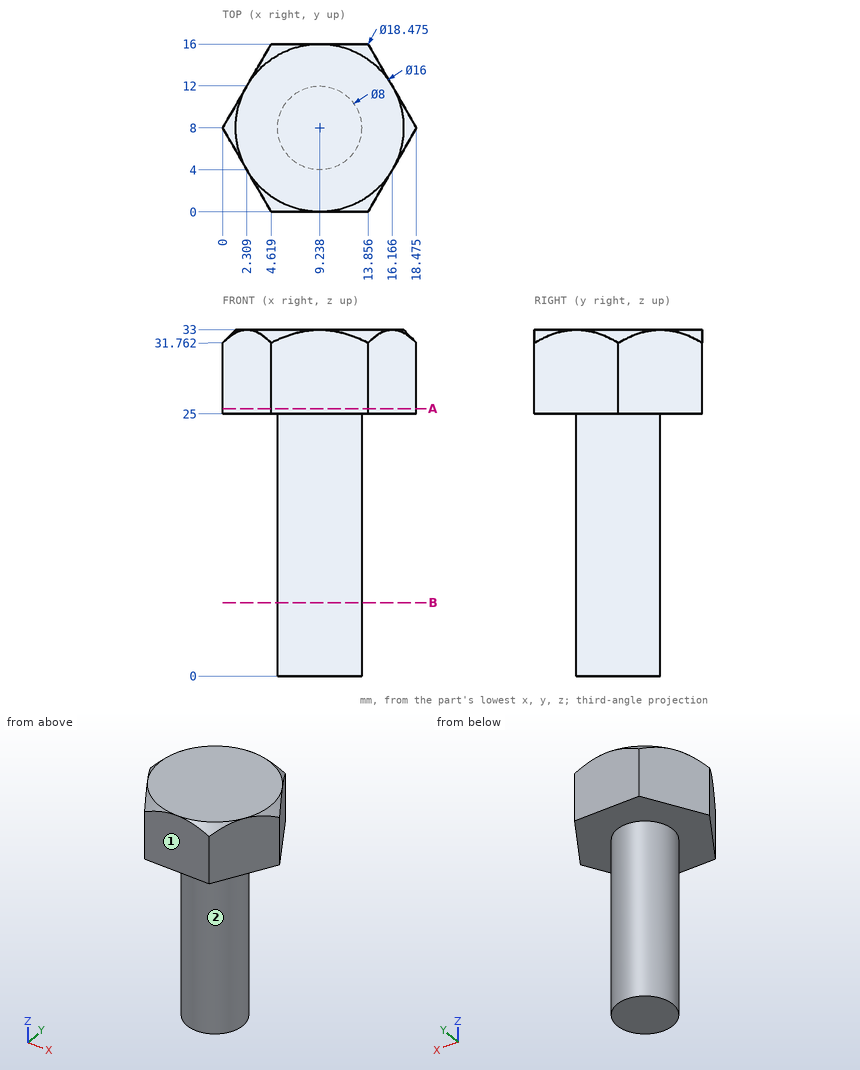
Input: dimensioned drawing with shaded views. Units: mm. Origin: part minimum x, y, z. A direction names the side the tool comes from. Coordinates: 2 decimals unless noted, no trailing zeros. Order: outer loops, then holes, each group sorted by start corner. A loop starts at its lowest first (then second) coordinate and runs counter-clockwise, first axis right, second up.
1. Cut plane B-B, the plane z = 7. Return loops of the section in (x, y).
Checked values:
outline: circle Ø8 at (9.24, 8)
2. Contact query for flat-ended pins moving along their axis: P1, Ø8, axis at y = 8.5, z = 27, coming from the -X side; P2, Ø6, axis at x = 2.5, y = 11.5, coming from the -Z side; P3, Ø2, axis at y = 4, z = 23.5, coming from the -X side; P4, Ø8, axis at y = 5.5, z = 11.5, coming from the +X side. Output: stop coordinate, or through.
Checked values:
P1: stops at x = 0
P2: stops at z = 25
P3: stops at x = 6.59
P4: stops at x = 13.24
3. Cut plane A-A, the plane z = 25.5. Return loops of the section in (x, y) (1 decimal).
Checked values:
outline: (0, 8) - (4.6, 0) - (13.9, 0) - (18.5, 8) - (13.9, 16) - (4.6, 16) - close
4. Access query for the marked faces 1 and 2. Directions: +Z, -Z, +X, -X, +Y, -Y. A direction counts if a zero-diameter tool reaches every point of the face in a straight line with its end or side. Return the directions, or none.
Checked values:
face 1: +Z, -Z, +X, -X, -Y
face 2: -Z
5. Ray query, line 1 along Z through (x, y) = (15.75, 7.25); line 2 along Y through (x, z) = (11.25, 14); line 3 along Y through (x, z) = (10.5, 21.5) (1 decimal). Return the intervals inside material, ascending.
Checked values:
line 1: z = 25 to 33
line 2: y = 4.54 to 11.46
line 3: y = 4.2 to 11.8
